Can you work these out from the model? Positions are in its coordinate system, mm. A direction names the side the tool comes from. Round coordinates to 2 decimals unless told otherwise and drop trailing zeros. Order: outer loops, then holes, each group sorted by start corner. A loop starts at its lowest first (then second) coordinate and runs counter-clockwise, first axis right, second up. Notation, with made-up numbers: (2, 59) -> (6, 59) arc R10 cw to (6, 64) -> close; hole circle Ø9 at (57.5, 23). An arc over 180 degrees is marked (long way). Use a Markdown table: item, result. Add a question column.
Q1. If we section it at C-C on x = -41.5: List the corners of the cut face in (y, z) for me, plus the area to 3 significant figures.
Q2. We'd pull the mould along X, two halves only. Please class faces 1 (the face through (37.5, -0.5, -33.8)), 2 (the face through (0, 0, -1.6)), 3 (the face through (49.787, -1.427, 11.056)): +X half, -X half, draft (parallel to the pull), parting line (faces both ways), or undercut.
Q3. If we section it at A-A on y = 1.25: List the corners of the cut face in (x, z) for me.
Q4. If we section it at B-B on z = 11: List the corners of the cut face in (x, y) for me (3 decimals), plus the area to 3 significant figures.
Q5. For faces 4 (the face through (11, 2.381, 1)), 5 (the face through (37.5, 0.5, -33.8)), 6 (the face through (-1.396, 0.033, 0.782)), which set-ups out of +Z, -Z, +X, -X, +Y, -Y let a thin tool reach every point of the face, with its end or its side?
Q6. I need wall thicknesses on line 1 along Z through (x, y) = (-5, -0.6); line 2 along X through (y, z) = (-0.85, -45); line 3 along Z through (x, y) = (-28, 1.7). Which ranges of each line are inside material? Lowest first, please. Write a range as [from, to].
Q7. I'm going to push flat-ended pins straight in: pin 1 Ø1.5 at (y, z) = (2, 28.5) entering from +X; pin 2 Ø1 at (x, y) = (-28, -2) entering from +Z; pin 3 Ø1.5 at (y, z) = (-1, -25) entering from +X. Where does each tip first touch, or does it pass through?
```python
from build123d import *

# Parameters (mm, degrees)
ESBO_O1_R                = 51
RESSALTO_EXTRUS_O1_DEPTH = 2.38125
ESBO_O2_R                = 51
ESBO_O2_R_2              = 50
CORTE_EXTRUS_O1_DEPTH    = 0.5
ESBO_O3_R                = 0.5
CORTE_EXTRUS_O2_DEPTH    = 1.88125
CORTE_EXTRUS_O3_DEPTH    = 73.281957681


with BuildPart() as part:
    # Esboço1 → Ressalto-extrusão1 (new, symmetric)
    with BuildSketch(Plane(origin=(0, 0, 0), x_dir=(1, 0, 0), z_dir=(0, 1, 0))):
        with Locations(Location((0, 0, 0), (0, 0, 90))):
            Circle(ESBO_O1_R)
    extrude(amount=RESSALTO_EXTRUS_O1_DEPTH, both=True)

    # Esboço2 → Corte-extrusão1 (cut, symmetric)
    with BuildSketch(Plane(origin=(0, 0, 0), x_dir=(1, 0, 0), z_dir=(0, 1, 0))):
        with Locations(Location((0, 0, 0), (0, 0, 90))):
            Circle(ESBO_O2_R)
        with Locations(Location((0, 0, 0), (0, 0, 270))):
            Circle(ESBO_O2_R_2, mode=Mode.SUBTRACT)
    extrude(amount=CORTE_EXTRUS_O1_DEPTH, both=True, mode=Mode.SUBTRACT)

    # Esboço3 → Corte-extrusão2 (cut)
    with BuildSketch(Plane(origin=(0, -0.5, 0), x_dir=(1, 0, 0), z_dir=(0, 1, 0))):
        with Locations(Location((0.789504293, -50, 0), (0, 0, 270))):
            Circle(ESBO_O3_R)
    extrude(amount=-CORTE_EXTRUS_O2_DEPTH, mode=Mode.SUBTRACT)

    # Esboço4 → Corte-extrusão3 (cut, through all)
    with BuildSketch(Plane(origin=(0, 2.38125, 0), x_dir=(1, 0, 0), z_dir=(0, 1, 0))):
        with BuildLine():
            Line((-2.14062409, 0.507669683), (-0.630657203, -2.107669683))
            ThreePointArc((-0.630657203, -2.107669683), (0, -2.2), (0.630657203, -2.107669683))
            Line((0.630657203, -2.107669683), (2.14062409, 0.507669683))
            ThreePointArc((2.14062409, 0.507669683), (1.905255888, 1.1), (1.509966887, 1.6))
            Line((1.509966887, 1.6), (-1.509966887, 1.6))
            ThreePointArc((-1.509966887, 1.6), (-1.905255888, 1.1), (-2.14062409, 0.507669683))
        make_face()
    extrude(amount=-CORTE_EXTRUS_O3_DEPTH, mode=Mode.SUBTRACT)


solid = part.part
```
Answer below:
| question | item | result |
|---|---|---|
| 1 | outline | (-2.38, -29.64) -> (-0.5, -29.64) -> (-0.5, -27.89) -> (0.5, -27.89) -> (0.5, -29.64) -> (2.38, -29.64) -> (2.38, 29.64) -> (0.5, 29.64) -> (0.5, 27.89) -> (-0.5, 27.89) -> (-0.5, 29.64) -> (-2.38, 29.64) -> close |
| 1 | area | 279 mm² |
| 2 | face 1 | draft |
| 2 | face 2 | undercut |
| 2 | face 3 | parting line |
| 3 | outline | circle Ø102 at (0, 0); hole (-2.14, -0.51) arc R2.2 ccw to (-1.51, -1.6) -> (1.51, -1.6) arc R2.2 ccw to (2.14, -0.51) -> (0.63, 2.11) arc R2.2 ccw to (-0.63, 2.11) -> close |
| 4 | outline | (-49.8, -2.381) -> (49.8, -2.381) -> (49.8, -0.5) -> (48.775, -0.5) -> (48.775, 0.5) -> (49.8, 0.5) -> (49.8, 2.381) -> (-49.8, 2.381) -> (-49.8, 0.5) -> (-48.775, 0.5) -> (-48.775, -0.5) -> (-49.8, -0.5) -> close |
| 4 | area | 472 mm² |
| 5 | face 4 | +Z, -Z, +X, -X, +Y |
| 5 | face 5 | none |
| 5 | face 6 | +Y, -Y |
| 6 | line 1 | [-50.75, 50.75] |
| 6 | line 2 | [-24, 24] |
| 6 | line 3 | [-42.63, 42.63] |
| 7 | pin 1 | x = 42.79 |
| 7 | pin 2 | z = 42.95 |
| 7 | pin 3 | x = 44.87 |
